```python
from build123d import *

# Parameters (mm, degrees)
BOSS_EXTRUDE1_DEPTH = 3


with BuildPart() as part:
    # Sketch1 → Boss-Extrude1 (new body)
    with BuildSketch(Plane(origin=(0, 0, 0), x_dir=(0, 0, -1), z_dir=(1, 0, 0))):
        Polygon((10, -3), (0, -3), (0, -8), (3, -8), (3, -13), (0, -13), (0, -18), (3, -18), (3, -23), (0, -23), (0, -28), (3, -28), (3, -33), (0, -33), (0, -38), (3, -38), (3, -43), (0, -43), (0, -48), (3, -48), (3, -48.75), (120, 0), (110, 0), (110, -3), (100, -3), (100, 0), (90, 0), (90, -3), (80, -3), (80, 0), (70, 0), (70, -3), (60, -3), (60, 0), (50, 0), (50, -3), (40, -3), (40, 0), (30, 0), (30, -3), (20, -3), (20, 0), (10, 0), align=None)
    extrude(amount=BOSS_EXTRUDE1_DEPTH)


solid = part.part
```
Design review of the part built by this model. Coordinates are the model's own, in mm. A direction names the side the tool comes from. Coordinates: 2 decimals unless noted, no trailing zeros. Loops run counter-clockwise (first coordinate to the right, second up) from the corner with the lowest first, then second, coordinate; pieces in that order, holes last.
Q1. Tool access review of faces 1 (the face through (1, -35, 0)), 2 (the face through (3, -19, -46)), 3 (the face through (1, -1, -110)), 4 (the face through (1, -3, -5)), 5 (the face through (1, -38, -1)): name each direction out of +Z, -Z, +X, -X, +Y, -Y from which nothing blocks a thin tool from reaching the whole face with its end or side.
Reported:
face 1: +Z, +X, -X, +Y, -Y
face 2: +Z, -Z, +X, +Y, -Y
face 3: +X, -X, +Y
face 4: +Z, +X, -X, +Y
face 5: +Z, +X, -X
Q2. We need section B-B on y = -35. State the section outline as (x, z) points.
Reported:
outline: (0, -36) - (3, -36) - (3, 0) - (0, 0) - close
Q3. To check wall thickness, follow line 1 (Z direction, x = 0.5, y = -25); line 2 (Y direction, x = 2.4, z = -111.5); line 3 (Z direction, x = 0.7, y = -44). State the ranges of each line that lie inside material, in increasing order.
Reported:
line 1: z = -60 to 0
line 2: y = -3.54 to 0
line 3: z = -14.4 to 0
Q4. For pin 1 (10 mm diameter, centred on y = -42, z = -45, fed in from -X); pin 2 (0.9 mm diameter, centred on x = 2, y = -1, fed in from -Z); pin 3 (2 mm diameter, centred on y = -22.5, z = -33.5, fed in from -X); pin 4 (0.9 mm diameter, centred on x = 1.5, z = -3.5, fed in from +Y), all flat-tipped, find the tip position at first contact; note any pin that passes through.
Reported:
pin 1: passes through
pin 2: stops at z = -118.68
pin 3: stops at x = 0
pin 4: stops at y = -3
Q5. We need section A-A on z = -42. State the section outline as (x, y) points, and give its area (3 significant figures).
Reported:
outline: (0, -32.5) - (3, -32.5) - (3, -3) - (0, -3) - close
area: 88.5 mm2
